The drawing under review shows one solid part. Ordinate dimensions are in mm from its lowest x, y, z. Coordinates: 2 decimals unless noted, no trailing zeros. Order: outer loops, then holes, each group sorted by start corner. A loop starts at its lowest first (then second) coordinate and runs counter-clockwise, first axis right, second up. Notation, with made-up numbers: (49, 80) -> (108, 80) arc R17 cw to (108, 102) -> close; hole circle Ø10 at (-17, 65.5). An arc over 180 degrees is marked (long way). Put each result on its own line as item: value.
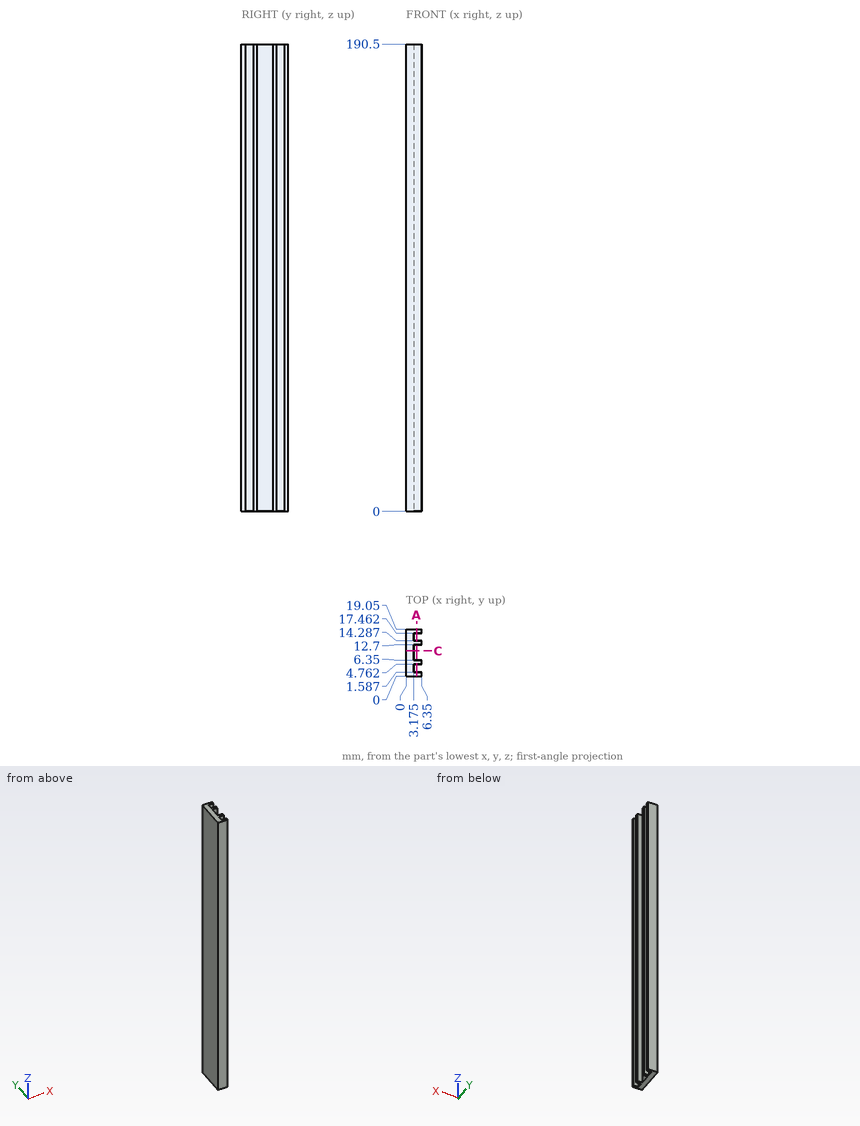
Item 1: For pin 1 Ø2.5 at (y, z) = (16, 137) entering from +X (1 decimal), flat-tipped, find the tip position at first contact; note if it passes through.
Answers below:
pin 1: x = 3.2
Item 2: Consider section A-A on x = 4.25. Write out the cut boundary in (y, z).
Answers below:
outline: (0, 0) -> (1.59, 0) -> (1.59, 190.5) -> (0, 190.5) -> close; (4.76, 0) -> (6.35, 0) -> (6.35, 190.5) -> (4.76, 190.5) -> close; (12.7, 0) -> (14.29, 0) -> (14.29, 190.5) -> (12.7, 190.5) -> close; (17.46, 0) -> (19.05, 0) -> (19.05, 190.5) -> (17.46, 190.5) -> close
Item 3: Consider section C-C on y = 10.25. Write out the cut boundary in (x, z) (1 decimal).
Answers below:
outline: (0, 0) -> (3.2, 0) -> (3.2, 190.5) -> (0, 190.5) -> close
Item 4: For line 1 (Y direction, x = 3.5, z = 28.5); line 2 (X direction, y = 9.5, z = 10.5) (1 decimal), list the stretches that pass through material, from the lowest coordinate up. Write a range as from..to.
Answers below:
line 1: 0..1.59, 4.76..6.35, 12.7..14.29, 17.46..19.05
line 2: 0..3.2
